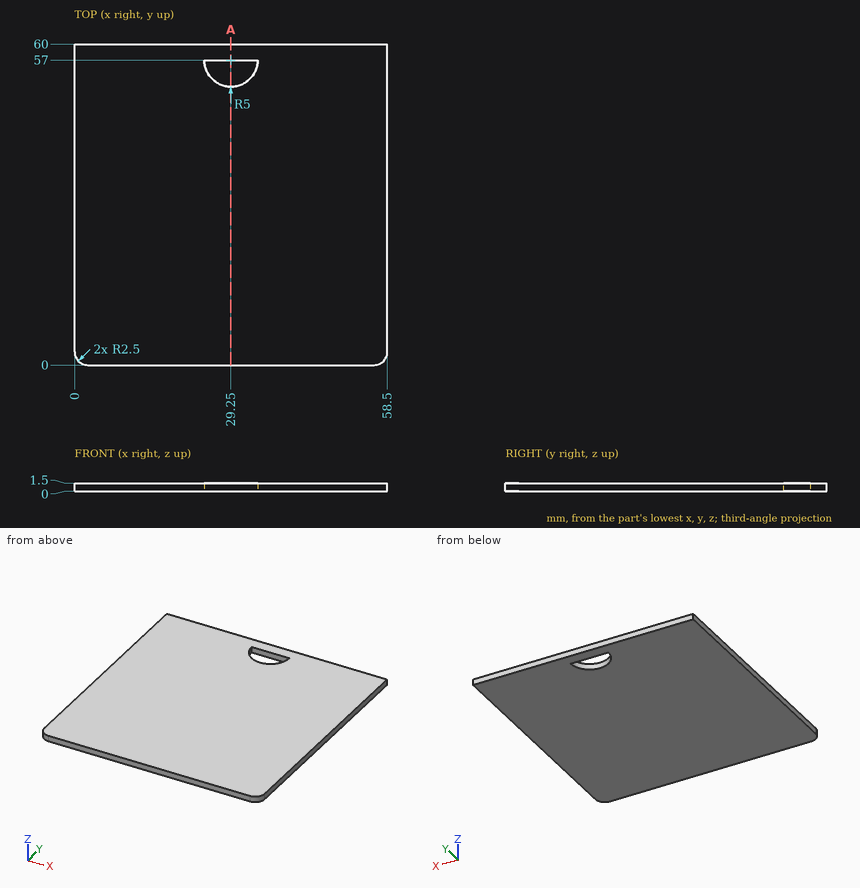
Geometry check sheet. Reference: drawing and pictorial views, mm from the part's lowest x, y, z. Give positions to 0.01 mm unless a question says otherwise; leave off trailing zeros. Order: outer loops, then holes, each group sorted by start corner. A loop starts at its lowest first (then second) coordinate and runs counter-clockwise, first axis right, second up. Notation, with made-up numbers: M 37.25,33 L 48.25,33 A17 cw 48.25,40 Z; hole C -9,-28.5 d7. An arc over 180 degrees is marked long. Answer in a Markdown table with one row per item. Add a question column.
Q1. Thickness scan on L1, parallel to Y at x = 26, z = 0.2; L2, parallel to Y at x = 33, z = 0.4; L3, parallel to X at y = 2, z = 0.75. Record the ranges inside material, lowest first.
Q2. Sectioned sample at A-A, the plane x = 29.25. Record the boundary of the cut face in (y, z), and give its area (3 significant figures).
Q3. Gauge pin test, flat end, axial feed: pin 1 Ø6 at (x, y) = (28.5, 30.5) entering from -Z. Record the tip position at first contact, or that the pin passes through.
Verdict:
| question | item | result |
|---|---|---|
| 1 | L1 | 0 to 53.2, 57 to 60 |
| 1 | L2 | 0 to 53.69, 57 to 60 |
| 1 | L3 | 0.05 to 58.45 |
| 2 | outline | M 0,0 L 52,0 L 52,1.5 L 0,1.5 Z; M 57,0 L 60,0 L 60,1.5 L 57,1.5 Z |
| 2 | area | 82.5 mm² |
| 3 | pin 1 | z = 0 |
